Source: CAD feature listing. Evaluate the final solid. Frame: model axes, mm. Face numbers are marked on the shaded views. A direction names the side the tool comes from. Give positions to 0.01 mm unless a question says otherwise; leave off trailing zeros. Loops run counter-clockwise (first coordinate to the right, second up) from the corner with the lowest first, then second, coordinate; pieces in that order, holes last.
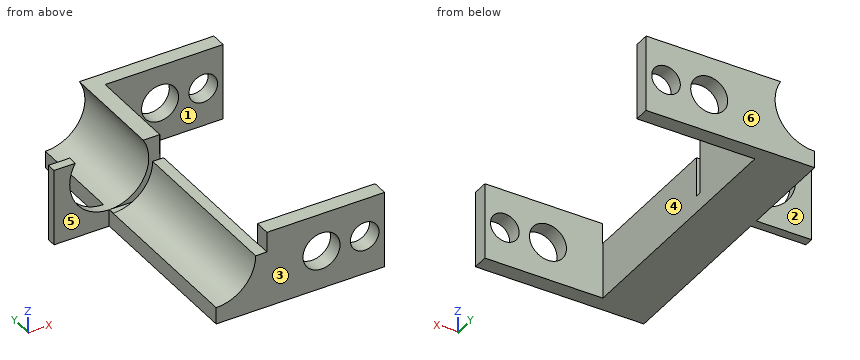
from build123d import *

# Parameters (mm, degrees)
SKETCH1_W              = 1526.54
SKETCH1_H              = 693.42
SKETCH1_R              = 129.54
SKETCH1_R_2            = 167.64
BOSS_EXTRUDE1_DEPTH    = 2540
SKETCH6_W              = 1068.621988509
SKETCH6_H              = 2260.925218267
CUT_EXTRUDE1_DEPTH     = 2540
CUT_EXTRUDE2_START     = -1590.133899231
CUT_EXTRUDE2_OUTLINE_W = 457.2
CUT_EXTRUDE2_OUTLINE_H = 182.88
CUT_EXTRUDE2_DEPTH     = 1590.133899231
SKETCH21_W             = 358.24
SKETCH21_H             = 57
CUT_EXTRUDE3_DEPTH     = 572.124
SKETCH22_W             = 693.42
SKETCH22_H             = 83.82
BOSS_EXTRUDE3_DEPTH    = 500.38
CUT_EXTRUDE4_DEPTH     = 2616.2
SKETCH24_R             = 358.25
CUT_EXTRUDE5_DEPTH     = 2616.2
SKETCH25_W             = 3.793020403
SKETCH25_H             = 182.88
CUT_EXTRUDE7_DEPTH     = 1590.294
SCALE1_SCALE           = 0.03937


# Read off the part's stored shape, not the designer's step: Cut-Extrude2
with BuildPart() as part:
    # Sketch1 → Boss-Extrude1 (new body)
    with BuildSketch(Plane(origin=(0, 0, 0), x_dir=(1, 0, 0), z_dir=(0, 1, 0))):
        with Locations((763.27, 346.71)):
            Rectangle(SKETCH1_W, SKETCH1_H)
        with Locations(Location((1346.125866933, 346.71, 0), (0, 0, 90))):
            Circle(SKETCH1_R, mode=Mode.SUBTRACT)
        with Locations(Location((954.97060339, 346.71, 0), (0, 0, 90))):
            Circle(SKETCH1_R_2, mode=Mode.SUBTRACT)
    extrude(amount=BOSS_EXTRUDE1_DEPTH)

    # Sketch6 → Cut-Extrude1 (cut)
    with BuildSketch(Plane.XY):
        with Locations((992.229005746, 1271.841969381)):
            Rectangle(SKETCH6_W, SKETCH6_H)
    extrude(amount=-CUT_EXTRUDE1_DEPTH, mode=Mode.SUBTRACT)

    # Cut-Extrude2 outline → Cut-Extrude2 (cut)
    with BuildSketch(Plane.XZ.offset(CUT_EXTRUDE2_START)):
        with Locations((228.6, -91.44)):
            Rectangle(CUT_EXTRUDE2_OUTLINE_W, CUT_EXTRUDE2_OUTLINE_H)
    extrude(amount=CUT_EXTRUDE2_DEPTH, mode=Mode.SUBTRACT)

    # Sketch21 → Cut-Extrude3 (cut)
    with BuildSketch(Plane.ZY):
        with Locations((-362, 1561.633899231)):
            Rectangle(SKETCH21_W, SKETCH21_H)
    extrude(amount=-CUT_EXTRUDE3_DEPTH, mode=Mode.SUBTRACT)

    # Sketch22 → Boss-Extrude3 (add)
    with BuildSketch(Plane.ZY):
        with Locations((-346.71, 1632.043899231)):
            Rectangle(SKETCH22_W, SKETCH22_H)
    extrude(amount=BOSS_EXTRUDE3_DEPTH)

    # Sketch23 → Cut-Extrude4 (cut)
    with BuildSketch(Plane.XZ):
        with BuildLine():
            Line((343.932135816, -182.88), (358.25, -182.88))
            ThreePointArc((358.25, -182.88), (-253.32100436, 70.44100436), (0, -541.13))
            Line((0, -541.13), (0, -182.88))
            Line((0, -182.88), (343.932135816, -182.88))
        make_face()
    extrude(amount=-CUT_EXTRUDE4_DEPTH, mode=Mode.SUBTRACT)

    # Sketch24 → Cut-Extrude5 (cut)
    with BuildSketch(Plane.XZ):
        with Locations((0, -182.88)):
            Circle(SKETCH24_R)
    extrude(amount=-CUT_EXTRUDE5_DEPTH, mode=Mode.SUBTRACT)

    # Sketch25 → Cut-Extrude7 (cut)
    with BuildSketch(Plane.XZ):
        with Locations((459.096510201, -91.44)):
            Rectangle(SKETCH25_W, SKETCH25_H)
    extrude(amount=-CUT_EXTRUDE7_DEPTH, mode=Mode.SUBTRACT)


with BuildPart() as part_1:
    # Scale1: scaled about (485.081829704, 1303.748157577, -445.917993823)
    add(part.part.scale(SCALE1_SCALE).moved(Location((465.984158069, 1252.419592613, -428.362202406))))


solid = part_1.part
1) Contact query for flat-ended pins moving along their axis: P1, Ø12, axis at x = 492.5, y = 1268.5, coming from the -Z side; P2, Ø6.5, axis at y = 1336, z = -452.5, coming from the -X side; P3, Ø5, axis at y = 1292.5, z = -437, coming from the -X side; P4, Ø13.5, axis at y = 1297, z = -447.5, coming from the +X side. Output: stop coordinate, or through.
Checks:
P1: passes through
P2: stops at x = 465.98
P3: stops at x = 479.53
P4: stops at x = 484.01
2) Reachability of the marked faces 1, 2 and 3 from +Z, -Z, +X, -X, +Y, -Y: full face, straight path, thin tool, end or side. Return the list, or none.
Checks:
face 1: +Z, -Z, +X
face 2: +Z, -Z, -X, +Y
face 3: +Z, -Z, +X, -X, -Y
3) Cut plane A-A (z = -440.5). State how many separate pieces and enclosed holes the cut face has, and give its area (3 significant figures).
Checks:
separate pieces: 7
enclosed holes: 0
area: 706 mm2
4) Pull-direction query (Y, two-part tool) for the marked faces 4, 5 and 6; classes: released by +Y, released by -Y, zero draft, split by the parting line, or undercut.
Checks:
face 4: undercut
face 5: released by -Y
face 6: released by +Y
5) Ray query, probe 1 along Y at (x, z) = (492, -447.75); probe 2 along X at (y, z) = (1288.5, -450.25); probe 3 along Y at (x, z) = (451, -432.5). Return the intervals inside material, ascending.
Checks:
probe 1: y = 1252.42 to 1257.99, 1347 to 1352.42
probe 2: x = 465.98 to 484.01
probe 3: y = 1315.02 to 1318.32
6) Cut plane C-C (y = 1288). Return loops of the section in (x, z), and give its area (3 significant figures).
Checks:
outline: (465.98, -455.66) - (484.01, -455.66) - (484.01, -435.56) - (480.09, -435.56) arc R14.1 cw to (465.98, -449.67) - close
area: 206 mm2
